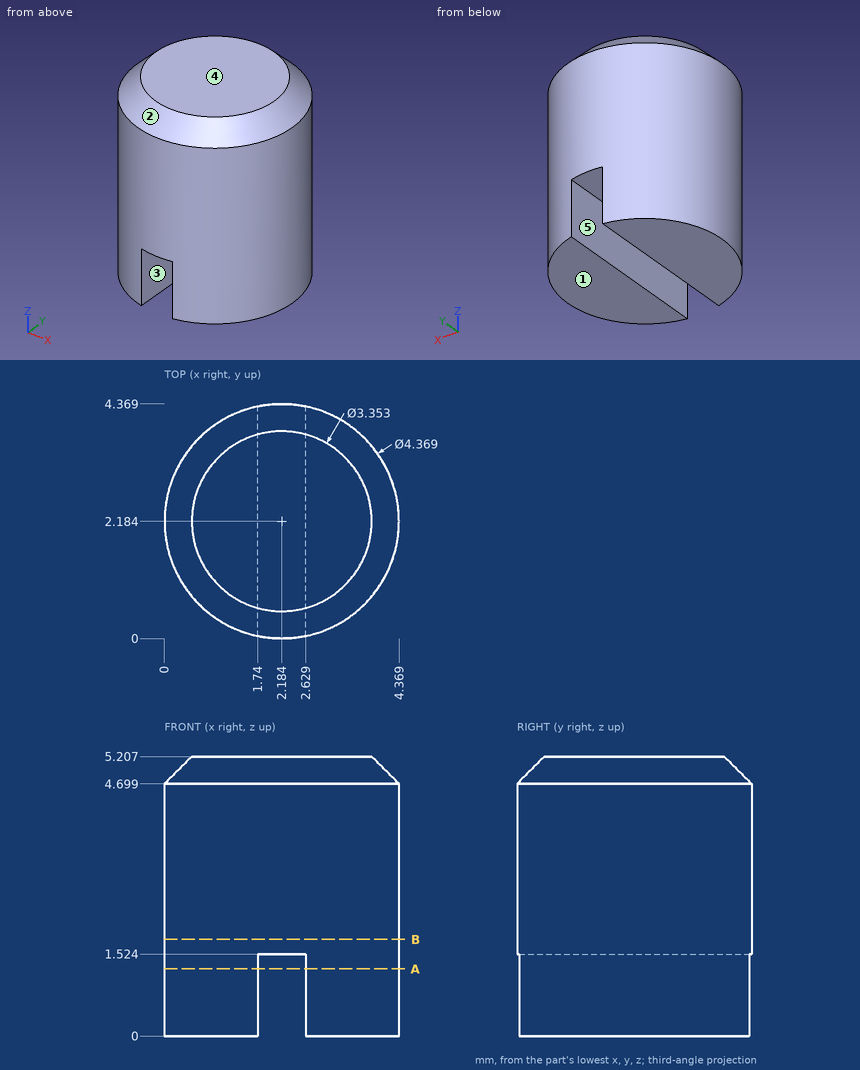
Could you check a few things on this drawing? It's one solid part, dimensions in mm from its lowest x, y, z. A direction names the side the tool comes from. Round coordinates to 2 decimals unless told otherwise and drop trailing zeros. Loops run counter-clockwise (first coordinate to the right, second up) from the corner with the lowest first, then second, coordinate; pieces in that order, holes last.
Q1. I want a section at A-A (z = 1.25). Write out the boundary of the cut face in (x, y) (1 decimal).
Q2. For P1, Ø0.8, axis at y = 1.5, z = 1, coming from the -X side, with a flat end and sliding along its axis, tell me the tip position at first contact or that it passes through.
Q3. I want a section at B-B (z = 1.8). Write out the boundary of the cut face in (x, y) (1 decimal), and give its area (3 significant figures).
Q4. Please list where these lines run through material, in increasing order: L1, parallel to X at y = 1.3, z = 1.25; L2, parallel to X at y = 0.3, z = 0.5; L3, parallel to Y at x = 4.15, z = 3.55 (1 decimal).
Q5. On a 3-axis mill with a long thin cutter (end or side, diameter ignored), from which of +Z, -Z, +X, -X, +Y, -Y can I reach the whole of each face in a straight line? I mean the marked faces 4 and 5. Say none if no direction works.
Q6. Thinking about a two-plate mould opening in X: for the marked faces 1, 2 and 3, which applies, pulls with the +X half, pulls with the -X half, needs draft (parallel to the pull), parting line crosses it, or undercut?
Answer below:
1. outline: (1.7, 0) - (1.7, 4.3) arc R2.2 ccw to start; (2.6, 0) arc R2.2 ccw to (2.6, 4.3) - close
2. P1: stops at x = 0.02
3. outline: circle Ø4.4 at (2.2, 2.2)
3. area: 15.0 mm2
4. L1: x = 0.19 to 1.74, 2.63 to 4.18
4. L2: x = 1.08 to 1.74, 2.63 to 3.29
4. L3: y = 1.2 to 3.1
5. face 4: +Z, +X, -X, +Y, -Y
5. face 5: -Z, +Y, -Y
6. face 1: needs draft
6. face 2: parting line crosses it
6. face 3: undercut
